Check sheet for the modelled part. Datum: model origin and axes. Units: mm. A direction names the side the tool comes from. Coordinates: 2 decimals unless noted, no trailing zeros. Loops run counter-clockwise (first coordinate to the right, second up) from the corner with the lowest first, then second, coordinate; pieces in that order, holes last. Notation, with made-up numbers: M 75,-21.75 L 101,-21.75 A16 cw 101,-16.75 Z; hole C -18.75,34 d4. An arc over 180 degrees is marked long. Use CSV: the item, a comma, the result in double quotes. Start each with the question number.
(1) Scan lines: line 1 (Y direction, x = -8, z = -3.8); line 2 (Y direction, x = -16.5, z = -0.45); line 3 (Y direction, x = -43, z = -4.65). Record each from-to range of solid material in increasing order.
(2) Draft check along Y on faces 3 (the flat face through (-19, 35, -5)), 4 (the flat face through (-8, 68.883, -2)), 5 (the flat face through (-25, 121.308, -2)). Enter one of: pulls with the +Y half, pulls with the -Y half, needs draft (parallel to the pull), parting line crosses it, or undercut.
(3) Go/stop test with a flat-tipped pin: pin 1 Ø1.6 at (y, z) = (2, -2) entering from +X. Record where the tip stops, or that it passes through.
(4) Section check D-D on x = -31. Record the cut outline in (y, z), and give its area (3 significant figures).
(5) Section check A-A on x = -7. Record the cut outline in (y, z), and give its area (3 significant figures).
(6) Section check B-B on x = -39. Record the cut outline in (y, z), and give its area (3 significant figures).
(7) Set-up check for faces 1 (the flat face through (-9, 63.733, -2)), 2 (the cylindrical face through (-2.72, -52.76, -2.46)): record each of +Z, -Z, +X, -X, +Y, -Y from which the full face is reachable in a straight line by a thin tool's end or side.
(8) Section check C-C on z = -1.7. Record the cut outline in (x, y), and give its area (3 significant figures).
from build123d import *

# Parameters (mm, degrees)
FLANGE_BASE1_DEPTH    = 5
CORTE_EXTRUS_O1_REACH = 132.145
ESBO_O2_R             = 1


# Sheet-metal steps are written as plain solids
with BuildPart() as part:
    # Esboço1 → Flange-base1 (new body)
    with BuildSketch(Plane.XY):
        with BuildLine():
            Line((-1.722631236, 117.808229797), (-1.722631236, 68.883230259))
            Line((-1.722631236, 68.883230259), (-16.138228035, 68.883230259))
            Line((-16.138228035, 68.883230259), (-16.138228035, 63.733230259))
            Line((-16.138228035, 63.733230259), (-1.722631236, 63.733230259))
            Line((-1.722631236, 63.733230259), (-1.722631236, 3.883229335))
            Line((-1.722631236, 3.883229335), (-16.138228035, 3.883229335))
            Line((-16.138228035, 3.883229335), (-16.138228035, -1.266770665))
            Line((-16.138228035, -1.266770665), (-1.722631236, -1.266770665))
            Line((-1.722631236, -1.266770665), (-1.722631236, -50.315698913))
            ThreePointArc((-1.722631236, -50.315698913), (-2.747757502, -52.790572648), (-5.222631236, -53.815698913))
            Line((-5.222631236, -53.815698913), (-43.33867275, -53.815698913))
            ThreePointArc((-43.33867275, -53.815698913), (-46.237739354, -52.276671331), (-46.587238264, -49.01307767))
            ThreePointArc((-46.587238264, -49.01307767), (-26.931743246, 33.601550332), (-46.499490821, 116.237005793))
            ThreePointArc((-46.499490821, 116.237005793), (-46.351024737, 119.645444535), (-43.371991, 121.308229797))
            Line((-43.371991, 121.308229797), (-5.222631236, 121.308229797))
            ThreePointArc((-5.222631236, 121.308229797), (-2.747757502, 120.283103531), (-1.722631236, 117.808229797))
        make_face()
    extrude(amount=-FLANGE_BASE1_DEPTH)

    # Esboço2 → Corte-extrusão1 (cut, up to next)
    with BuildSketch(Plane.XY, mode=Mode.PRIVATE) as corte_extrus_o1_sk1:
        with Locations((-16.138228035, 68.883230259)):
            Circle(ESBO_O2_R)
    corte_extrus_o1_tool1 = extrude(corte_extrus_o1_sk1.sketch, amount=-CORTE_EXTRUS_O1_REACH, mode=Mode.PRIVATE) & part.part
    # Esboço2 → Corte-extrusão1 (cut, up to next)
    with BuildSketch(Plane.XY, mode=Mode.PRIVATE) as corte_extrus_o1_sk2:
        with Locations((-16.138228035, 63.733230259)):
            Circle(ESBO_O2_R)
    corte_extrus_o1_tool2 = extrude(corte_extrus_o1_sk2.sketch, amount=-CORTE_EXTRUS_O1_REACH, mode=Mode.PRIVATE) & part.part
    # Esboço2 → Corte-extrusão1 (cut, up to next)
    with BuildSketch(Plane.XY, mode=Mode.PRIVATE) as corte_extrus_o1_sk3:
        with Locations((-16.138228035, 3.883229335)):
            Circle(ESBO_O2_R)
    corte_extrus_o1_tool3 = extrude(corte_extrus_o1_sk3.sketch, amount=-CORTE_EXTRUS_O1_REACH, mode=Mode.PRIVATE) & part.part
    # Esboço2 → Corte-extrusão1 (cut, up to next)
    with BuildSketch(Plane.XY, mode=Mode.PRIVATE) as corte_extrus_o1_sk4:
        with Locations((-16.138228035, -1.266770665)):
            Circle(ESBO_O2_R)
    corte_extrus_o1_tool4 = extrude(corte_extrus_o1_sk4.sketch, amount=-CORTE_EXTRUS_O1_REACH, mode=Mode.PRIVATE) & part.part
    add(corte_extrus_o1_tool1.solids().sort_by_distance((-16.138228, 68.88323, 0))[0], mode=Mode.SUBTRACT)
    add(corte_extrus_o1_tool2.solids().sort_by_distance((-16.138228, 63.73323, 0))[0], mode=Mode.SUBTRACT)
    add(corte_extrus_o1_tool3.solids().sort_by_distance((-16.138228, 3.883229, 0))[0], mode=Mode.SUBTRACT)
    add(corte_extrus_o1_tool4.solids().sort_by_distance((-16.138228, -1.266771, 0))[0], mode=Mode.SUBTRACT)


solid = part.part
Outcome:
1,line 1,"y = -53.82 to -1.27, 3.88 to 63.73, 68.88 to 121.31"
1,line 2,"y = -53.82 to -2.2, -0.33 to 2.95, 4.82 to 62.8, 64.67 to 67.95, 69.82 to 121.31"
1,line 3,"y = -53.82 to -41.47, 108.87 to 121.31"
2,face 3,"needs draft"
2,face 4,"undercut"
2,face 5,"pulls with the +Y half"
3,pin 1,"stops at x = -16.14"
4,outline,"M -53.82,-5 L -4.76,-5 L -4.76,0 L -53.82,0 Z; M 72.16,-5 L 121.31,-5 L 121.31,0 L 72.16,0 Z"
4,area,"491 mm²"
5,outline,"M -53.82,-5 L -1.27,-5 L -1.27,0 L -53.82,0 Z; M 3.88,-5 L 63.73,-5 L 63.73,0 L 3.88,0 Z; M 68.88,-5 L 121.31,-5 L 121.31,0 L 68.88,0 Z"
5,area,"824 mm²"
6,outline,"M -53.82,-5 L -31.81,-5 L -31.81,0 L -53.82,0 Z; M 99.21,-5 L 121.31,-5 L 121.31,0 L 99.21,0 Z"
6,area,"220 mm²"
7,face 1,"+Z, -Z, +X"
7,face 2,"+Z, -Z, +X, -Y"
8,outline,"M -46.59,-49.01 A3.5 ccw -43.34,-53.82 L -5.22,-53.82 A3.5 ccw -1.72,-50.32 L -1.72,-1.27 L -15.14,-1.27 A1 cw long -16.14,-0.27 L -16.14,2.88 A1 cw long -15.14,3.88 L -1.72,3.88 L -1.72,63.73 L -15.14,63.73 A1 cw long -16.14,64.73 L -16.14,67.88 A1 cw long -15.14,68.88 L -1.72,68.88 L -1.72,117.81 A3.5 ccw -5.22,121.31 L -43.37,121.31 A3.5 ccw -46.5,116.24 A183.86 cw Z"
8,area,"5,500 mm²"
